```python
from build123d import *

# Parameters (mm, degrees)
PAD_DEPTH       = 27
POCKET_DEPTH    = 18
PAD001_DEPTH    = 5
POCKET001_DEPTH = 8


with BuildPart() as part:
    # Sketch → Pad (new body)
    with BuildSketch(Plane.XY):
        Polygon((-20.307119, 40.133461), (19.519873, 40.133461), (30.657932, 19.882448), (20.194906, 0), (20.194906, -19.944538), (-20.307119, -19.944538), (-20.307119, 0), (-30.432625, 20.219969), align=None)
    extrude(amount=PAD_DEPTH)

    # Sketch001 (on Face10 of Pad) → Pocket (cut)
    with BuildSketch(Plane.XY.offset(27)):
        Polygon((-14.705877, -3.167421), (-10.180991, -3.393665), (-10.63348, -16.289593), (-14.705877, -16.515837), align=None)
        Polygon((-5.203616, -2.968245), (0, -3.167421), (0, -15.15837), (-5.203616, -15.15837), align=None)
        Polygon((3.167424, -3.393665), (7.46607, -3.393665), (7.013581, -15.15837), (2.488694, -14.932126), align=None)
        Polygon((10.859732, -4.751131), (16.063354, -4.751131), (16.063354, -16.968325), (10.407243, -16.742081), align=None)
    extrude(amount=-POCKET_DEPTH, mode=Mode.SUBTRACT)

    # Sketch002 (on Face5 of Pocket) → Pad001 (join)
    with BuildSketch(Plane.XY.offset(27)):
        Polygon((0, 21.168507), (-5.353663, 14.129646), (5.389863, 14.129646), align=None)
    extrude(amount=PAD001_DEPTH)

    # Sketch003 (on Face5 of Pad001) → Pocket001 (cut)
    with BuildSketch(Plane.XY.offset(27)):
        Polygon((-12.432311, 32.022194), (-19.256838, 26.107605), (-6.821035, 26.107605), align=None)
        Polygon((12.014428, 31.966341), (5.341558, 26.051752), (18.838953, 26.051752), align=None)
    extrude(amount=-POCKET001_DEPTH, mode=Mode.SUBTRACT)


solid = part.part
```
Geometry: final body of the model. Coordinates: model frame, mm. A direction names the side the tool comes from. Round coordinates to 2 decimals unless told otherwise and drop trailing zeros. Order: outer loops, then holes, each group sorted by start corner. A loop starts at its lowest first (then second) coordinate and runs counter-clockwise, first axis right, second up. Notation, with made-up numbers: (-4.5, 20.5) - (21.5, 20.5) arc R19 cw to (21.5, 56.5) - close; hole circle Ø4 at (79, 25). An arc over 180 degrees is marked (long way). Use CSV: the item, a comma, the result in double quotes. Start each with the question number.
Q1. Section query B-B (x = -2.5). Return loops of the section in (y, z), and give its area (3 significant figures).
Q2. Section query D-D (z = 6.5). Return loops of the section in (x, y).
Q3. Section query A-A (z = 20). State how many separate pieces and enclosed holes the cut face has, and give its area (3 significant figures).
Q4. First-contact query: pin 1 (10 mm diameter, centred on x = 11, y = 33.5, fed in from +Z); pin 2 (1.5 mm diameter, centred on x = 0, z = 28.5, fed in from -Y); pin 3 (6 mm diameter, centred on y = -10.5, z = 16, fed in from +X). Flat tips, straight axial feed; report the tip coordinate or a pass-through.
Q5. Section query C-C (y = 18). Return loops of the section in (x, z).
Q6. Access query for faces 5 (the face through (-2.638, -3.066, 18.126)), 6 (the face through (20.195, -10, 13)). Directions: +Z, -Z, +X, -X, +Y, -Y. A direction counts if a zero-diameter tool reaches every point of the face in a straight line with its end or side. Return the directions, or none.
Q7. Mould query, pull axis Y, two halves, no side actions, for faces 1 (the face through (-20.307, -10, 13)), 2 (the face through (0, 14.13, 29)), 3 (the face through (-1, 40.133, 13)), 4 (the face through (-3, -9, 9)). Classes: +Y half, -Y half, draft (parallel to the pull), parting line (faces both ways), or undercut.
Q8. Material intervals for line 1 along Y through (x, z) = (-5, 20); line 2 along X through (y, z) = (-12, 3.5); line 3 along Z through (x, y) = (-27.5, 17.5), sorted ascending. Write a range as from..to.
Result set:
1,outline,"(-19.94, 0) - (40.13, 0) - (40.13, 27) - (17.88, 27) - (17.88, 32) - (14.13, 32) - (14.13, 27) - (-3.07, 27) - (-3.07, 9) - (-15.16, 9) - (-15.16, 27) - (-19.94, 27) - close"
1,area,"1,420 mm2"
2,outline,"(-30.43, 20.22) - (-20.31, 0) - (-20.31, -19.94) - (20.19, -19.94) - (20.19, 0) - (30.66, 19.88) - (19.52, 40.13) - (-20.31, 40.13) - close"
3,separate pieces,"1"
3,enclosed holes,"6"
3,area,"2,530 mm2"
4,pin 1,"stops at z = 27"
4,pin 2,"stops at y = 14.13"
4,pin 3,"stops at x = 20.19"
5,outline,"(-29.32, 0) - (29.67, 0) - (29.67, 27) - (2.43, 27) - (2.43, 32) - (-2.41, 32) - (-2.41, 27) - (-29.32, 27) - close"
6,face 5,"+Z"
6,face 6,"+Z, -Z, +X, -Y"
7,face 1,"draft"
7,face 2,"-Y half"
7,face 3,"+Y half"
7,face 4,"undercut"
8,line 1,"y = -19.94..-15.16, -2.98..40.13"
8,line 2,"x = -20.31..20.19"
8,line 3,"z = 0..27"
